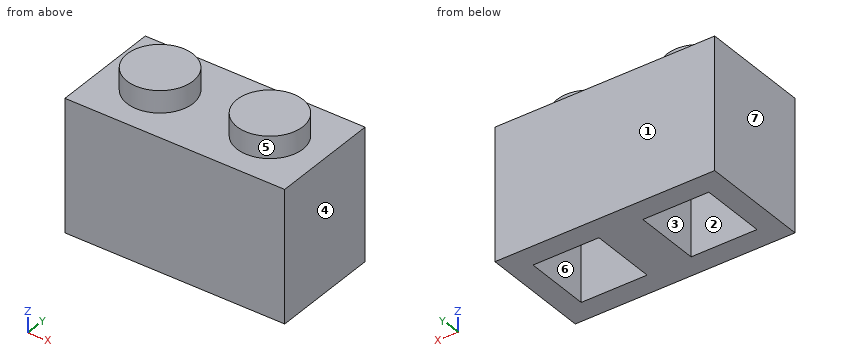
from build123d import *

# Parameters (mm, degrees)
F0_W     = 16
F0_H     = 8
F0_W_2   = 4.8
F0_H_2   = 4.8
F0_W_3   = 3.2
F1_DEPTH = 9.6
F2_DEPTH = 8
F3_DEPTH = 9.6
F4_R     = 1.6
F5_DEPTH = 1.6
F6_R     = 2.4
F6_R_2   = 1.6
F7_DEPTH = 1.6


with BuildPart() as f1:
    # F0 (on Top) → F1 (new body)
    with BuildSketch(Plane.XY):
        Rectangle(F0_W, F0_H)
        Polygon((-1.6, -2.4), (-6.4, -2.4), (-6.4, 2.4), (-1.6, 2.4), (1.6, 2.4), (6.4, 2.4), (6.4, -2.4), (1.6, -2.4), align=None, mode=Mode.SUBTRACT)
        with Locations((-4, 0)):
            Rectangle(F0_W_2, F0_H_2)
        Rectangle(F0_W_3, F0_H_2)
        with Locations((4, 0)):
            Rectangle(F0_W_2, F0_H_2)
    extrude(amount=F1_DEPTH)

    # F0 (on Top) → F2 (cut)
    with BuildSketch(Plane.XY):
        with Locations((-4, 0)):
            Rectangle(F0_W_2, F0_H_2)
        Rectangle(F0_W_3, F0_H_2)
        with Locations((4, 0)):
            Rectangle(F0_W_2, F0_H_2)
    extrude(amount=F2_DEPTH, mode=Mode.SUBTRACT)

    # F0 (on Top) → F3 (join)
    with BuildSketch(Plane.XY):
        Rectangle(F0_W_3, F0_H_2)
    extrude(amount=F3_DEPTH)

    # F4 (on face) → F5 (cut)
    with BuildSketch(Plane.XY.offset(9.6)):
        with Locations((-4, 0)):
            Circle(F4_R)
        with Locations((4, 0)):
            Circle(F4_R)
    extrude(amount=-F5_DEPTH, mode=Mode.SUBTRACT)

    # F6 (on face) → F7 (join)
    with BuildSketch(Plane.XY.offset(9.6)):
        with Locations((-4, 0)):
            Circle(F6_R)
        with Locations((-4, 0)):
            Circle(F6_R_2, mode=Mode.SUBTRACT)
        with Locations((4, 0)):
            Circle(F6_R)
        with Locations((4, 0)):
            Circle(F6_R_2, mode=Mode.SUBTRACT)
        with Locations((-4, 0)):
            Circle(F6_R_2)
        with Locations((4, 0)):
            Circle(F6_R_2)
    extrude(amount=F7_DEPTH)


solid = f1.part
The model under review builds one solid part; all positions refer to its coordinate system, in mm. Face numbers are marked on the shaded views. A direction names the side the tool comes from. Round coordinates to 2 decimals unless told otherwise and drop trailing zeros. Loops run counter-clockwise (first coordinate to the right, second up) from the corner with the lowest first, then second, coordinate; pieces in that order, holes last. Notation, with made-up numbers: M 88.5,-22.5 L 147.5,-22.5 A17 cw 147.5,-9.5 Z; hole C 3,23.25 d11. An arc over 180 degrees is marked long. Answer as a JSON object with one key per item and string values.
Item 1: Tool access review of the marked faces 5, 6 and 7: name each direction out of +Z, -Z, +X, -X, +Y, -Y from which nothing blocks a thin tool from reaching the whole face with its end or side.
Check sheet entries:
{"face 5": "+Z", "face 6": "-Z", "face 7": "+Z, -Z, -X, +Y, -Y"}
Item 2: We need section C-C, the plane x = -4. State the section outline as (y, z) points.
Check sheet entries:
{"outline": "M -4,0 L -2.4,0 L -2.4,8 L -1.6,8 L -1.6,9.6 L 1.6,9.6 L 1.6,8 L 2.4,8 L 2.4,0 L 4,0 L 4,9.6 L 2.4,9.6 L 2.4,11.2 L -2.4,11.2 L -2.4,9.6 L -4,9.6 Z"}
Item 3: Clearance check with flat-ended pins moving along their axes: P1, Ø1.9, axis at x = -4, y = 0, coming from the -Z side; P2, Ø4, axis at x = 4, y = 0, coming from the -Z side. State where each tip first meets the part, or that it passes through.
Check sheet entries:
{"P1": "z = 9.6", "P2": "z = 8"}
Item 4: We need section A-A, the plane z = 2. State the section outline as (x, y) points, and give its area (3 significant figures).
Check sheet entries:
{"outline": "M -8,-4 L 8,-4 L 8,4 L -8,4 Z; hole M -6.4,-2.4 L -1.6,-2.4 L -1.6,2.4 L -6.4,2.4 Z; hole M 1.6,-2.4 L 6.4,-2.4 L 6.4,2.4 L 1.6,2.4 Z", "area": "81.9 mm2"}
Item 5: The part is to be moulded in two halves that separate along Y. For the marked faces 1, 2, 3 and 4, say which applies: +Y half, -Y half, draft (parallel to the pull), parting line (faces both ways), or undercut.
Check sheet entries:
{"face 1": "+Y half", "face 2": "undercut", "face 3": "undercut", "face 4": "draft"}
Item 6: We need section D-D, the plane z = 8.75. State the section outline as (x, y) points, and give its area (3 significant figures).
Check sheet entries:
{"outline": "M -8,-4 L 8,-4 L 8,4 L -8,4 Z; hole C -4,0 d3.2; hole C 4,0 d3.2", "area": "112 mm2"}
Item 7: For line 1 along X through (y, z) = (0.75, 2.25); line 2 along Y through (x, z) = (-4.75, 2.5); line 3 along Y through (x, z) = (-4, 9.25), list the stretches that pass through material, from the lowest coordinate up.
Check sheet entries:
{"line 1": "-8 to -6.4, -1.6 to 1.6, 6.4 to 8", "line 2": "-4 to -2.4, 2.4 to 4", "line 3": "-4 to -1.6, 1.6 to 4"}
Item 8: We need section B-B, the plane y = 0. State the section outline as (x, z) points.
Check sheet entries:
{"outline": "M -8,0 L -6.4,0 L -6.4,8 L -5.6,8 L -5.6,9.6 L -2.4,9.6 L -2.4,8 L -1.6,8 L -1.6,0 L 1.6,0 L 1.6,8 L 2.4,8 L 2.4,9.6 L 5.6,9.6 L 5.6,8 L 6.4,8 L 6.4,0 L 8,0 L 8,9.6 L 6.4,9.6 L 6.4,11.2 L 1.6,11.2 L 1.6,9.6 L -1.6,9.6 L -1.6,11.2 L -6.4,11.2 L -6.4,9.6 L -8,9.6 Z"}
